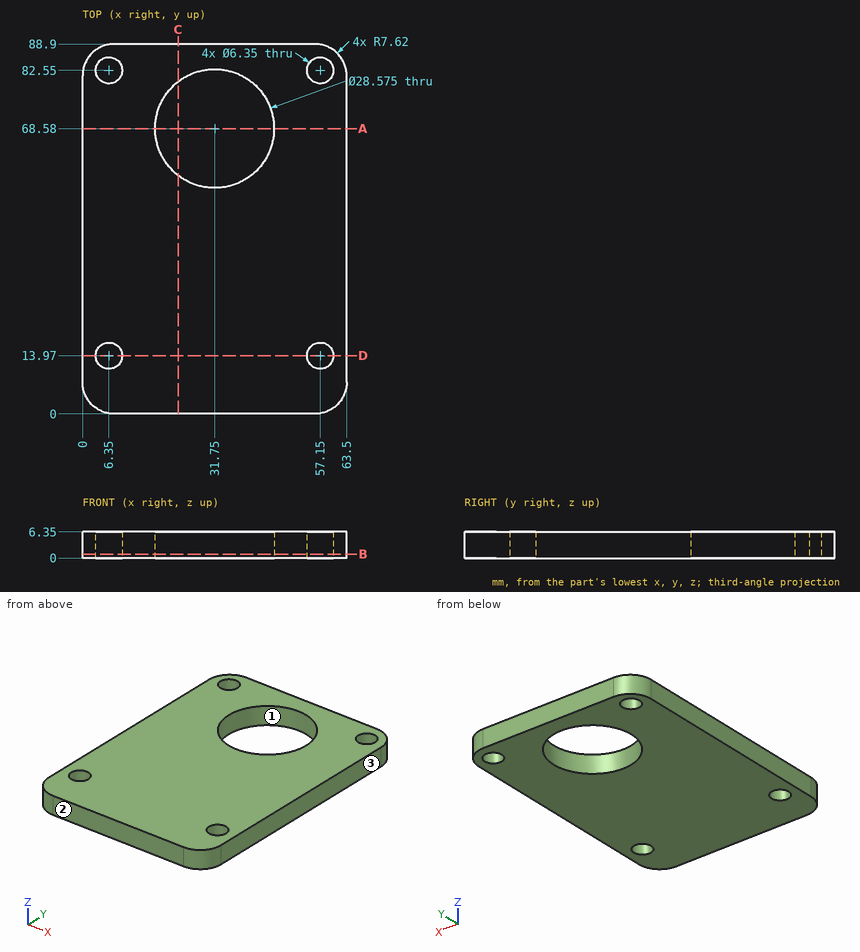
Could you check a few things on this drawing? It's one solid part, dimensions in mm from its lowest x, y, z. Give positions to 0.01 mm unless a question says otherwise; leave off trailing zeros. Write each loop counter-clockwise with the first axis right and the second up, starting at its lowest first coordinate (ties: lowest second). Pieces come first, ordered by that corner, then holes. Notation, with made-up numbers: (-28.5, 14.25) -> (-12.5, 14.25) arc R12 ccw to (-12.5, 32.25) -> close; hole circle Ø5 at (-39.75, 88.25). An arc over 180 degrees is marked (long way). Answer as CSV lines item,"result". Start each with the question number.
(1) If we section it at B-B, the plane z = 1: Give the number of separate pieces and of enclosed holes in the cut face, and give its area (3 significant figures).
(2) Please list where these lines run through material, in increasing order: line 1 (Y direction, x = 4.5, z = 5); line 2 (Y direction, x = 6.35, z = 5) (3 decimals); line 3 (Y direction, x = 25, z = 4.5).
(3) If we section it at A-A, the plane y = 68.58: Write out the boundary of the cut face in (x, z).
(4) If we section it at C-C, the plane x = 23: Write out the boundary of the cut face in (y, z).
(5) I'm going to push a flat-ended pin straight in: pin 1 Ø5 at (x, y) = (6.35, 13.97) entering from +Z. Where does the tip first touch, or does it pass through?
(6) If we mould it in two halves opening along X, with no side actions, what happens to the marked faces 1, 2 and 3? For each: +X half, -X half, draft (parallel to the pull), parting line (faces both ways), or undercut.
(7) If we section it at D-D, the plane y = 13.97: Write out the boundary of the cut face in (x, z) (3 decimals), and give its area (3 significant figures).
Answer list:
1,separate pieces,"1"
1,enclosed holes,"5"
1,area,"4,830 mm^2"
2,line 1,"0.67 to 11.39, 16.55 to 79.97, 85.13 to 88.23"
2,line 2,"0.107 to 10.795, 17.145 to 79.375, 85.725 to 88.793"
2,line 3,"0 to 55.99, 81.17 to 88.9"
3,outline,"(0, 0) -> (17.46, 0) -> (17.46, 6.35) -> (0, 6.35) -> close; (46.04, 0) -> (63.5, 0) -> (63.5, 6.35) -> (46.04, 6.35) -> close"
4,outline,"(0, 0) -> (57.29, 0) -> (57.29, 6.35) -> (0, 6.35) -> close; (79.87, 0) -> (88.9, 0) -> (88.9, 6.35) -> (79.87, 6.35) -> close"
5,pin 1,"through"
6,face 1,"undercut"
6,face 2,"draft"
6,face 3,"+X half"
7,outline,"(0, 0) -> (3.175, 0) -> (3.175, 6.35) -> (0, 6.35) -> close; (9.525, 0) -> (53.975, 0) -> (53.975, 6.35) -> (9.525, 6.35) -> close; (60.325, 0) -> (63.5, 0) -> (63.5, 6.35) -> (60.325, 6.35) -> close"
7,area,"323 mm^2"
